```python
from build123d import *

# Parameters (mm, degrees)
EXTRUDE_1_DEPTH = 80
EXTRUDE_START   = 5
EXTRUDE_2_DEPTH = 5


with BuildPart() as part:
    # 草圖1 → 填料-伸長1 (new body)
    with BuildSketch(Plane.XY):
        with BuildLine():
            Line((0, -37), (0, -40))
            ThreePointArc((0, -40), (20, 34.641016151), (-34.641016151, -20))
            Line((-34.641016151, -20), (-32.04293994, -18.5))
            ThreePointArc((-32.04293994, -18.5), (18.5, 32.04293994), (0, -37))
        make_face()
    extrude(amount=EXTRUDE_1_DEPTH)

    # 草圖2 → 填料-伸長2 (add)
    with BuildSketch(Plane(origin=(0, 0, 0), x_dir=(-1, 0, 0), z_dir=(0, 0, -1)).offset(EXTRUDE_START)):
        with BuildLine():
            Line((0, -30), (0, -40))
            ThreePointArc((0, -40), (-38.14867803, -12.02823198), (-22.943057454, 32.766081772))
            Line((-22.943057454, 32.766081772), (-17.207293091, 24.574561329))
            ThreePointArc((-17.207293091, 24.574561329), (-28.611508522, -9.021173985), (0, -30))
        make_face()
    extrude(amount=-EXTRUDE_2_DEPTH)


solid = part.part
```
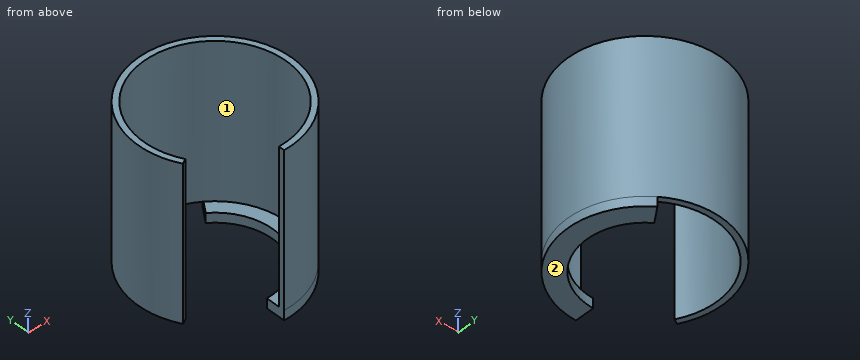
Can you work these out from the model? Positions are in its coordinate system, mm. Face numbers are marked on the shaded views. Give positions to 0.01 mm unless a question says otherwise; leave off trailing zeros. Order: outer loops, then holes, each group sorted by start corner. A loop starts at its lowest first (then second) coordinate and runs counter-clockwise, first axis right, second up. Notation, with made-up numbers: M 25.5,51 L 37.5,51 A13 cw 37.5,67 Z; hole C -13.5,63 d5. An arc over 180 degrees is marked long. Write item = value, one per line. Start each with the question number.
Q1. I need wall thicknesses on probe 1 along X at (y, z) = (0, 56); probe 2 along Y at (x, z) = (1, 11); probe 3 along Z at (x, y) = (27.5, -16.5). Which ranges of each line are inside material? Lowest first, please. Write a range as [from, to].
Q2. Suppose I cut it at A-A (y = 0). Write out the boundary of the cut face in (x, z).
Q3. Will these pins go through, and if not, where does the flat tip stop? pin 1 Ø5 at (y, z) = (-35.5, 36.5) entering from -X; pin 2 Ø4 at (y, z) = (-18.5, 38) entering from -X; pin 3 Ø4 at (x, z) = (-9, 69.5) entering from +Y.
Q4. We'd pull the mould along X, two halves only. Please class the marked faces 1 and 2: pulls with the +X half, pulls with the -X half, needs draft (parallel to the pull), parting line crosses it, or undercut.
Q5. Suppose I cut it at D-D (x = 26). Write out the boundary of the cut face in (y, z), plus the area to 3 significant figures.
Q6. Suppose I cut it at C-C (y = -35). Write out the boundary of the cut face in (x, z), plus the area to 3 significant figures.
Q7. Suppose I cut it at B-B (x = 12.5). Write out the boundary of the cut face in (y, z).
Check result:
q1.probe_1 = [-40, -37], [37, 40]
q1.probe_2 = [-39.99, -36.99], [36.99, 39.99]
q1.probe_3 = [-5, 0]
q2.outline = M -40,0 L -37,0 L -37,80 L -40,80 Z; M 30,-5 L 40,-5 L 40,80 L 37,80 L 37,0 L 30,0 Z
q3.pin_1 = 0
q3.pin_2 = -36.44
q3.pin_3 = 39.38
q4.face_1 = undercut
q4.face_2 = needs draft
q5.outline = M -30.4,-5 L -14.97,-5 L -14.97,0 L -26.32,0 L -26.32,80 L -30.4,80 Z; M 14.97,-5 L 30.4,-5 L 30.4,80 L 26.32,80 L 26.32,0 L 14.97,0 Z
q5.area = 806 mm2
q6.outline = M 0,-5 L 19.36,-5 L 19.36,80 L 12,80 L 12,0 L 0,0 Z
q6.area = 686 mm2
q7.outline = M -38,-5 L -27.27,-5 L -27.27,0 L -34.82,0 L -34.82,80 L -38,80 Z; M 34.82,0 L 38,0 L 38,80 L 34.82,80 Z
